For this review, take the finished solid that the model builds, in its own axes (mm). Face numbers are marked on the shaded views. A direction names the side the tool comes from. Round coordinates to 2 decimals unless told otherwise and drop trailing zeros. Order: outer loops, then holes, each group sorted by start corner. A loop starts at its lowest first (then second) coordinate and runs counter-clockwise, first axis right, second up. Notation, with made-up numbers: M 81.5,59.5 L 125.5,59.5 A14 cw 125.5,67.5 Z; hole C 56.25,66 d5. An arc over 180 degrees is marked long. Put each result on its own line as item: value.
from build123d import *

# Parameters (mm, degrees)
F0_W     = 45.2
F0_H     = 45.2
F0_W_2   = 41.2
F0_H_2   = 41.2
F1_DEPTH = 21
F2_SIZE  = 2


with BuildPart() as f1:
    # F0 (on Top) → F1 (new body)
    with BuildSketch(Plane.XY):
        Rectangle(F0_W, F0_H)
        Rectangle(F0_W_2, F0_H_2, mode=Mode.SUBTRACT)
    extrude(amount=F1_DEPTH)

    # F2
    f2_edges = [f1.edges().sort_by_distance(p)[0] for p in [
        (-22.6, -22.6, 10.5),
        (-20.6, -20.6, 10.5),
        (22.6, -22.6, 10.5),
        (20.6, -20.6, 10.5),
        (20.6, 20.6, 10.5),
        (-20.6, 20.6, 10.5),
        (22.6, 22.6, 10.5),
        (-22.6, 22.6, 10.5),
    ]]
    chamfer(f2_edges, length=F2_SIZE)


solid = f1.part
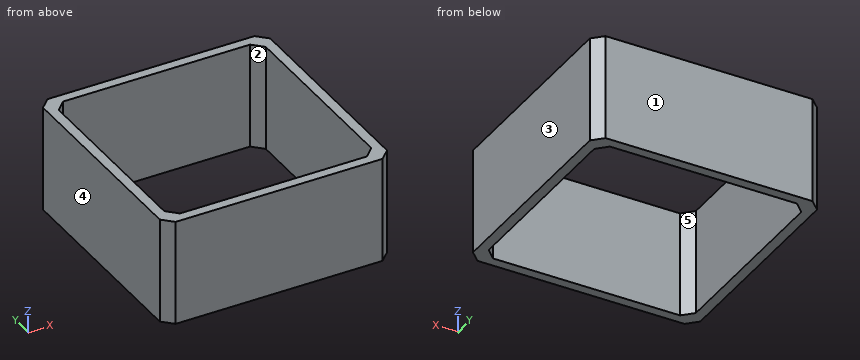
(1) To check wall thickness, follow L1, parallel to Y at x = 5, z = 16.75. State the ranges of the line that lie inside material, in increasing order.
A:
L1: y = -22.6 to -20.6, 20.6 to 22.6
(2) Add section B-B on z = 14. Give the boundary of the cut face in (x, y), then the cut area to 3 significant figures.
A:
outline: M -22.6,-20.6 L -20.6,-22.6 L 20.6,-22.6 L 22.6,-20.6 L 22.6,20.6 L 20.6,22.6 L -20.6,22.6 L -22.6,20.6 Z; hole M -20.6,-18.6 L -18.6,-20.6 L 18.6,-20.6 L 20.6,-18.6 L 20.6,18.6 L 18.6,20.6 L -18.6,20.6 L -20.6,18.6 Z
area: 346 mm2
(3) For the marked faces 4 and 5, list the 3-axis set-ups (+Z, -Z, +X, -X, +Y, -Y) from which the entire face can be reached by the end or side of a thin tool; tool diameter is ignored.
A:
face 4: +Z, -Z, -X, +Y, -Y
face 5: +Z, -Z
(4) Add section A-A on x = 12. Give the boundary of the cut face in (y, z).
A:
outline: M -22.6,0 L -20.6,0 L -20.6,21 L -22.6,21 Z; M 20.6,0 L 22.6,0 L 22.6,21 L 20.6,21 Z
(5) Draft analysis for pull direction X (two halves, no side actions). For the marked faces 1, 2 and 3, state which applies: released by +X, released by -X, zero draft, split by the parting line, or undercut.
A:
face 1: zero draft
face 2: undercut
face 3: released by +X
